Read the model definition and answer for the solid it produces. Units are mm, in the model's axes. A direction names the side the tool comes from. Round coordinates to 2 decimals unless told otherwise and drop trailing zeros. Order: outer loops, then holes, each group sorted by start corner. A loop starts at its lowest first (then second) coordinate and runs counter-clockwise, first axis right, second up. Notation, with made-up numbers: (49, 83) - (85, 83) arc R9 cw to (85, 88) - close; hole circle Ø9 at (-9.75, 41.25). An arc over 180 degrees is marked (long way). Answer as a JSON object with one key per item and string values. Group by question number.
Q1. Given pin 1 Ø10 at (y, z) = (70, 7.5) entering from +X; pin 2 Ø0.9 at (x, z) = (32, 10) entering from -Y; pin 3 Ø0.9 at (x, z) = (32, 10) entering from +Y, each flat-ended and moving along its own axis, determine where each tip first touches the part or whether it passes through.
Q2. The mould has two halves that part along Y. Classify faces 5 (the flat face through (-15, 119.182, 11)), 6 (the flat face through (30.926, 34.5, 7.6)), 7 (the flat face through (33, 45.682, 10)): pulls with the +Y half, pulls with the -Y half, needs draft (parallel to the pull), parting line crosses it, or undercut.
Q3. A cutting plane is placed at A-A on z = 4.75. Determine the outline of the cut face in (x, y).
Q4. A cutting plane is placed at C-C on y = 61. Determine the outline of the cut face in (x, z).
Q5. Consider line 1 (Y direction, x = -26, z = 2.25); line 2 (X direction, y = -39, z = 5.25); line 3 (Z direction, x = -31.5, y = 85). Determine where each line is inside the solid, lowest interval first.
Q6. A tool of negligible diameter and unlimited length cuts with its end or side. For faces 1 (the flat face through (-15, 37, 0)), 2 (the flat face through (35.3, 35.6, 8)), 3 (the flat face through (32, 44.682, 9)), 4 (the flat face through (29.426, 35, 11)), from which of +Z, -Z, +X, -X, +Y, -Y can it reach the whole face along a straight path? Write none if from no direction.
Q7. A cutting plane is placed at B-B on x = 18.5. Determine the outline of the cut face in (y, z).
```python
from build123d import *

# Parameters (mm, degrees)
F0_W         = 90
F0_H         = 170
F0_W_2       = 87
F0_H_2       = 167
F1_DEPTH     = 20
F2_DEPTH     = 2
F4_DEPTH     = 5
F5_T         = 1
F5_T3_DEPTH  = 6
F5_T5_DEPTH  = 22
F5_T7_DEPTH  = 89
F5_T9_DEPTH  = 20
F5_T11_DEPTH = 169
F6_T4_DEPTH  = 29.5866302263
F6_T6_DEPTH  = 44.819347292


# Not quite as in the source:
# - a fillet or chamfer that OpenCascade refuses, or shapes differently, is made with other operations: its cross-section is extruded or revolved along the edge and cut away or added
# - a shell that OpenCascade refuses in one call is made with other operations: the cavity is built on its own and cut out


with BuildPart() as f1:
    # F0 (on Top) → F1 (new body)
    with BuildSketch(Plane.XY):
        with Locations((-14.0737314522, 35.681976974)):
            Rectangle(F0_W, F0_H)
        with Locations((-14.0737314522, 35.681976974)):
            Rectangle(F0_W_2, F0_H_2, mode=Mode.SUBTRACT)
    extrude(amount=F1_DEPTH)

    # F0 (on Top) → F2 (join)
    with BuildSketch(Plane.XY):
        with Locations((-14.0737314522, 35.681976974)):
            Rectangle(F0_W_2, F0_H_2)
    extrude(amount=F2_DEPTH)

    # F3 (on face) → F4 (join)
    with BuildSketch(Plane.YZ.offset(30.9262685478)):
        Polygon((45.681976974, 12), (35.681976974, 12), (25.681976974, 12), (25.681976974, 8), (45.681976974, 8), align=None)
    extrude(amount=F4_DEPTH)

    # F5: shell of thickness 1, made by hand


with BuildPart() as f5_core1:
    # F5_t2: copy of F1
    add(f1.part)

    # the walls: a layer under each face that stays
    f5_faces = [f5_core1.faces().sort_by_distance(p)[0] for p in [
        (30.9262685478, -20.9846896927, 16.6666666667),
        (-14.0737314522, -49.318023026, 10),
        (-14.0737314522, 35.681976974, 0),
        (-57.6674814522, 85.0029646283, 20),
        (-14.0737314522, 120.681976974, 10),
        (33.4262685478, 45.681976974, 10),
        (33.4262685478, 25.681976974, 10),
        (33.4262685478, 35.681976974, 12),
        (-59.0737314522, 35.681976974, 10),
        (-14.0737314522, -47.818023026, 11),
        (-57.5737314522, 35.681976974, 11),
        (-14.0737314522, 119.181976974, 11),
        (29.4262685478, 35.681976974, 11),
        (35.9262685478, 35.681976974, 10),
        (-14.0737314522, 35.681976974, 2),
    ]]
    thicken(f5_faces, amount=-F5_T, mode=Mode.SUBTRACT)

    # F5_s4 → F5_t3 (cut)
    with BuildSketch(Plane.XY.offset(7)):
        Polygon((30.9362685478, 45.691976974), (29.9262685478, 45.681976974), (29.9262685478, 44.681976974), (30.9262685478, 44.681976974), align=None)
        Polygon((30.9362685478, 25.671976974), (29.9262685478, 25.681976974), (29.9262685478, 26.681976974), (30.9262685478, 26.681976974), align=None)
    extrude(amount=F5_T3_DEPTH, mode=Mode.SUBTRACT)

    # F5_s6 → F5_t5 (cut)
    with BuildSketch(Plane.XZ.offset(-46.681976974)):
        Polygon((30.9362685478, 12.01), (29.9262685478, 12), (29.9262685478, 11), (30.9262685478, 11), align=None)
    extrude(amount=F5_T5_DEPTH, mode=Mode.SUBTRACT)

    # F5_s8 → F5_t7 (cut)
    with BuildSketch(Plane.YZ.offset(-58.5737314522)):
        Polygon((-47.808023026, 2.01), (-48.818023026, 2), (-48.818023026, 1), (-47.818023026, 1), align=None)
        Polygon((119.171976974, 2.01), (120.181976974, 2), (120.181976974, 1), (119.181976974, 1), align=None)
    extrude(amount=F5_T7_DEPTH, mode=Mode.SUBTRACT)

    # F5_s10 → F5_t9 (cut)
    with BuildSketch(Plane.XY.offset(1)):
        Polygon((-57.5637314522, -47.808023026), (-57.5737314522, -48.818023026), (-58.5737314522, -48.818023026), (-58.5737314522, -47.818023026), align=None)
        Polygon((29.4162685478, -47.808023026), (29.4262685478, -48.818023026), (30.4262685478, -48.818023026), (30.4262685478, -47.818023026), align=None)
        Polygon((-57.5637314522, 119.171976974), (-58.5737314522, 119.181976974), (-58.5737314522, 120.181976974), (-57.5737314522, 120.181976974), align=None)
        Polygon((29.4162685478, 119.171976974), (29.4262685478, 120.181976974), (30.4262685478, 120.181976974), (30.4262685478, 119.181976974), align=None)
    extrude(amount=F5_T9_DEPTH, mode=Mode.SUBTRACT)

    # F5_s12 → F5_t11 (cut)
    with BuildSketch(Plane.XZ.offset(-120.181976974)):
        Polygon((-57.5637314522, 2.01), (-58.5737314522, 2), (-58.5737314522, 1), (-57.5737314522, 1), align=None)
        Polygon((29.4162685478, 2.01), (30.4262685478, 2), (30.4262685478, 1), (29.4262685478, 1), align=None)
    extrude(amount=F5_T11_DEPTH, mode=Mode.SUBTRACT)


with BuildPart() as f1_1:
    add(f1.part)

    # what is left inside the walls is the cavity
    f5_cavity = [f5_core1.part.solids().sort_by_distance(p)[0] for p in [
        (32.676269, 32.681977, 8.01),
    ]]
    add(f5_cavity, mode=Mode.SUBTRACT)

    # F6: fillet of radius 5.08 on 5 edges, made by hand


with BuildPart() as f6_tool2:
    # F6_s3 → F6_t4 (new body)
    with BuildSketch(Plane.XZ.offset(-56.2686072003)):
        with BuildLine():
            ThreePointArc((34.9262685478, 8), (33.0520512056, 10.1845515591), (30.2916164573, 11))
            Line((30.2916164573, 11), (34.9262685478, 11))
            Line((34.9262685478, 11), (34.9262685478, 8))
        make_face()
    extrude(amount=F6_T4_DEPTH)

    split(bisect_by=Plane.XZ.offset(-45.681976974), keep=Keep.TOP)


with BuildPart() as f1_2:
    add(f1_1.part)

    # F6_t1: union F6_tool2
    add(f6_tool2.part)

    # F6_s7 → F6_t6 (cut)
    with BuildSketch(Plane.XZ.offset(-58.09165062)):
        with BuildLine():
            ThreePointArc((35.9262685478, 8), (34.1498745795, 10.8755530587), (30.9623990894, 12))
            Line((30.9623990894, 12), (35.9262685478, 12))
            Line((35.9262685478, 12), (35.9262685478, 8))
        make_face()
    extrude(amount=F6_T6_DEPTH, mode=Mode.SUBTRACT)


solid = f1_2.part
```
Result set:
{
 "1": {"pin 1": "stops at x = 30.93", "pin 2": "stops at y = 25.68", "pin 3": "stops at y = 45.68"},
 "2": {"face 5": "undercut", "face 6": "needs draft", "face 7": "pulls with the +Y half"},
 "3": {"outline": "(-59.07, -49.32) - (30.93, -49.32) - (30.93, 120.68) - (-59.07, 120.68) - close; hole (-57.57, -47.82) - (29.43, -47.82) - (29.43, 119.18) - (-57.57, 119.18) - close"},
 "4": {"outline": "(-59.07, 0) - (30.93, 0) - (30.93, 20) - (29.43, 20) - (29.43, 2) - (-57.57, 2) - (-57.57, 20) - (-59.07, 20) - close"},
 "5": {"line 1": "y = -49.32 to -47.82, 119.18 to 120.68", "line 2": "x = -59.07 to -57.57, 29.43 to 30.93", "line 3": "z = 0 to 2"},
 "6": {"face 1": "-Z, +X, -X, +Y, -Y", "face 2": "-Z, +X, +Y, -Y", "face 3": "none", "face 4": "+Z"},
 "7": {"outline": "(-49.32, 0) - (120.68, 0) - (120.68, 20) - (119.18, 20) - (119.18, 2) - (-47.82, 2) - (-47.82, 20) - (-49.32, 20) - close"}
}
